Verification items for the finished model (mm, model axes). A direction names the side the tool comes from. Coordinates: 2 decimals unless noted, no trailing zeros. Loops run counter-clockwise (first coordinate to the right, second up) from the corner with the lowest first, then second, coordinate; pieces in that order, holes last.
Q1. Access from +Z, -Z, +X, -X, +Y, -Y to the whole of each face (thin tool, end or side, straight path). Record for faces 1 (the face through (142.434, -0.462, -23.565)), 2 (the face through (163, -26.386, -41)), 3 (the face through (159.163, -3.455, -12.677)).
Q2. Go/stop test with flat-tipped pins: P1, Ø6, axis at x = 180, z = -49.5, coming from the +Y side; P2, Ø10, axis at y = 13, z = -49, coming from the -X side; P3, Ø1.5, axis at x = 162.5, y = -22.5, coming from the +Z side; P4, Ø8, axis at y = 14, z = -14.5, coming from the -X side. Record where each tip stops, or that it passes through.
Q3. Sectioned sample at A-A (z = -30). Enter the section's corners in (x, y), then the cut area to 3 significant figures.
Q4. Material ranges on probe 1 along Z at (x, y) = (184, -2); probe 2 along X at (y, z) = (-19.5, -24); probe 3 along X at (y, z) = (16.5, -54.5), recorded low to high.
Q5. Sectioned sample at D-D (x = 151). Enter the section's corners in (y, z).
Q6. Sectioned sample at C-C (z = -22.5). Enter the section's corners in (x, y).
Q7. Sectioned sample at B-B (y = -8). Enter the section's corners in (x, z).
Q8. Mould release check, pull along X, two halves, no side actions. Record for faces 4 (the face through (148, -15, -41)), 5 (the face through (178.039, 14.785, -41.38)), 6 (the face through (141, 0, -26.1)): +X half, -X half, draft (parallel to the pull), parting line (faces both ways), or undercut.
```python
from build123d import *

# Parameters (mm, degrees)
SKETCH076_W             = 42.3
SKETCH076_H             = 42.3
PAD024_DEPTH            = 40
SKETCH075_R             = 11
PAD025_DEPTH            = 3
SKETCH077_R             = 5.1
PAD026_DEPTH            = 21
SKETCH079_R             = 1.5
POCKET047_DEPTH         = 5
CHAMFER008_SIZE         = 5
SKETCH080_R             = 6.75
PAD027_DEPTH            = 10
BODY017_PLACEMENT_ANGLE = 45


with BuildPart() as part:
    # Sketch076 → Pad024 (new body)
    with BuildSketch(Plane.XY):
        Rectangle(SKETCH076_W, SKETCH076_H)
    extrude(amount=PAD024_DEPTH)

    # Sketch075 (on Face6 of Pad024) → Pad025 (join)
    with BuildSketch(Plane.XY.offset(40)):
        Circle(SKETCH075_R)
    extrude(amount=PAD025_DEPTH)

    # Sketch077 (on Face8 of Pad025) → Pad026 (join)
    with BuildSketch(Plane.XY.offset(43)):
        Circle(SKETCH077_R)
    extrude(amount=PAD026_DEPTH)

    # Sketch079 (on Face5 of Pad026) → Pocket047 (cut)
    with BuildSketch(Plane.XY.offset(40)):
        with Locations((-15.5, 15.5)):
            Circle(SKETCH079_R)
        with Locations((15.5, 15.5)):
            Circle(SKETCH079_R)
        with Locations((15.5, -15.5)):
            Circle(SKETCH079_R)
        with Locations((-15.5, -15.5)):
            Circle(SKETCH079_R)
    extrude(amount=-POCKET047_DEPTH, mode=Mode.SUBTRACT)

    # Chamfer008
    chamfer008_edges = [part.edges().sort_by_distance(p)[0] for p in [
        (21.15, 21.15, 20),
        (21.15, -21.15, 20),
        (-21.15, 21.15, 20),
        (-21.15, -21.15, 20),
    ]]
    chamfer(chamfer008_edges, length=CHAMFER008_SIZE)

    # Sketch080 (on Face22 of Chamfer008) → Pad027 (join)
    with BuildSketch(Plane.XY.offset(64)):
        Circle(SKETCH080_R)
    extrude(amount=-PAD027_DEPTH)


with BuildPart() as part_1:
    # Body017 placement: moved
    add(part.part.moved(Location((162.9239407719, -0.0108408296, -61.1))).rotate(Axis((162.9239407719, -0.0108408296, -61.1), (0, 0, 1)), BODY017_PLACEMENT_ANGLE))


solid = part_1.part
```
Geometry check:
1. face 1: +Z
1. face 2: +Z, -Z, +X, -X, -Y
1. face 3: none
2. P1: stops at y = 15.82
2. P2: stops at x = 141.02
2. P3: stops at z = -26.1
2. P4: passes through
3. outline: (136.55, -3.55) - (159.39, -26.39) - (166.46, -26.39) - (189.3, -3.55) - (189.3, 3.52) - (166.46, 26.36) - (159.39, 26.36) - (136.55, 3.52) - close
3. area: 1,740 mm2
4. probe 1: z = -61.1 to -21.1
4. probe 2: x = 152.5 to 173.35
4. probe 3: x = 149.52 to 176.32
5. outline: (-18, -61.1) - (17.98, -61.1) - (17.98, -21.1) - (-18, -21.1) - close
6. outline: (136.55, -3.55) - (159.39, -26.39) - (166.46, -26.39) - (189.3, -3.55) - (189.3, 3.52) - (166.46, 26.36) - (159.39, 26.36) - (136.55, 3.52) - close; hole circle Ø3 at (141, -0.01); hole circle Ø3 at (162.92, -21.93); hole circle Ø3 at (162.92, 21.91); hole circle Ø3 at (184.84, -0.01)
7. outline: (141, -61.1) - (184.85, -61.1) - (184.85, -21.1) - (170.49, -21.1) - (170.49, -18.1) - (155.36, -18.1) - (155.36, -21.1) - (141, -21.1) - close
8. face 4: -X half
8. face 5: +X half
8. face 6: undercut
